from build123d import *

# Parameters (mm, degrees)
BOSS_EXTRUDE2_DEPTH                           = 9
CUT_EXTRUDE3_DEPTH                            = 37.794697197
CUT_EXTRUDE3_DEPTH_BACK                       = 29.526
SKETCH3_W                                     = 7.1119396
SKETCH3_H                                     = 8
SKETCH3_W_2                                   = 47.10835744
BOSS_EXTRUDE3_DEPTH                           = 14.032
BOSS_EXTRUDE3_DEPTH_BACK                      = 1
BOSS_EXTRUDE4_START                           = 2.072367721
BOSS_EXTRUDE4_DEPTH                           = 6.927632279
CSK_FOR_3_FLAT_HEAD_SOCKET_CAP_SCREW1_A_COUNT = 2
CSK_FOR_3_FLAT_HEAD_SOCKET_CAP_SCREW1_A_PITCH = 19.290792


# Read off the part's stored shape, not the designer's step: Boss-Extrude4
with BuildPart() as part:
    # Sketch2 → Boss-Extrude2 (new body)
    with BuildSketch(Plane.XY):
        Polygon((-9.096510891, -26.330282843), (-9.701316376, -34.435752293), (-2.609093023, -34.964952435), (-3.061940834, -41.033918716), (-2.048641284, -41.109525962), (-1.973042695, -40.096342438), (0.937582862, -1.088781958), (1.013181451, -0.075598434), (0, 0), (-0.567761002, -7.60900747), (-7.660098307, -7.079798826), (-8.264903605, -15.18526578), (-1.1725663, -15.714474425), (-2.004173586, -26.859491487), align=None)
    extrude(amount=BOSS_EXTRUDE2_DEPTH)

    # Sketch3 → Cut-Extrude3 (cut, two sides: drawn at the far end of the back side and taken through both)
    with BuildSketch(Plane(origin=(-2.608979071, -34.964960937, 0), x_dir=(0.9972277257028987, -0.07441010072177218, 0), z_dir=(-0.07441010072177218, -0.9972277257028987, 0)).offset(-CUT_EXTRUDE3_DEPTH_BACK)):
        with Locations((-3.556084069, 5)):
            Rectangle(SKETCH3_W, SKETCH3_H)
        with Locations((-30.666232589, 5)):
            Rectangle(SKETCH3_W_2, SKETCH3_H)
    extrude(amount=CUT_EXTRUDE3_DEPTH + CUT_EXTRUDE3_DEPTH_BACK, mode=Mode.SUBTRACT)

    # Sketch4 → Boss-Extrude3 (add, two sides: drawn at the far end of the back side and taken through both)
    with BuildSketch(Plane(origin=(1.013183369, -0.075600662, 0), x_dir=(0, 0, -1), z_dir=(0.9972277257028997, -0.07441010072175744, 0)).offset(-BOSS_EXTRUDE3_DEPTH_BACK)):
        Polygon((-9, -41.147998684), (-9, 2.079e-06), (-10, 0), (-10, -41.147998684), align=None)
    extrude(amount=BOSS_EXTRUDE3_DEPTH + BOSS_EXTRUDE3_DEPTH_BACK)

    # Boss-Extrude4 outline → Boss-Extrude4 (add)
    with BuildSketch(Plane.XY.offset(BOSS_EXTRUDE4_START)):
        Polygon((-0.054187906, -41.258346009), (3.007638975, -0.22441879), (1.013181451, -0.075598434), (0.937582862, -1.088781958), (-1.973042695, -40.096342438), (-2.048641284, -41.109525962), align=None)
    extrude(amount=BOSS_EXTRUDE4_DEPTH)

    # Sketch6 → CSK for _3 Flat Head Socket Cap Screw1 (revolve, cut)
    with BuildSketch(Plane(origin=(-4.41257913, -11.346475453, 1), x_dir=(0, -1, 0), z_dir=(1, 0, 0))):
        Polygon((0, 0), (0, 1), (1.397, 1), (1.397, 1.694722738), (2.8702, 0), align=None)
    csk_for_3_flat_head_socket_cap_screw1 = revolve(axis=Axis((-4.41257913, -11.346475453, 7.35), (0, 0, -1)), mode=Mode.SUBTRACT)

    # CSK for _3 Flat Head Socket Cap Screw1 a: CSK for _3 Flat Head Socket Cap Screw1 ×2
    with Locations(*[Vector(-0.07441010072177331, -0.9972277257028986, 0) * (i * CSK_FOR_3_FLAT_HEAD_SOCKET_CAP_SCREW1_A_PITCH) for i in range(1, CSK_FOR_3_FLAT_HEAD_SOCKET_CAP_SCREW1_A_COUNT)]):
        add(csk_for_3_flat_head_socket_cap_screw1, mode=Mode.SUBTRACT)


solid = part.part
Build history of the part. All positions in model axes, mm. A direction names the side the tool comes from. Coordinates: 2 decimals unless noted, no trailing zeros. Order: outer loops, then holes, each group sorted by start corner. A loop starts at its lowest first (then second) coordinate and runs counter-clockwise, first axis right, second up. Notation, with made-up numbers: (71, 4.5) - (96, 4.5) arc R15 cw to (96, 33.5) - close; hole circle Ø7 at (27.25, 36.5). An arc over 180 degrees is marked (long way). Put each result on its own line as item: value.
1. Probe line 1 along Z through (x, y) = (8.5, -9); line 2 along Y through (x, z) = (-6.5, 0.5); line 3 along X through (y, z) = (-8, 4.25). List the from-to ranges inside material, lowest first. Write a range as [from, to].
Answer sheet:
line 1: z = [9, 10]
line 2: y = [-34.67, -32.93], [-28.24, -26.52], [-15.32, -12.6], [-10.09, -7.17]
line 3: x = [-0.6, 2.43]
2. Saw through at D-D (x = 13). Write the cut outline in (y, z).
Answer sheet:
outline: (-28.01, 9) - (-0.97, 9) - (-0.97, 10) - (-28.01, 10) - close
3. Drop flat-ended pins along their axis: P1, Ø4, axis at x = -0.5, y = -11, coming from the -Z side; P2, Ø3, axis at y = -10, z = 9, coming from the -X side; P3, Ø1.5, axis at y = -37.5, z = 2.5, coming from the -X side; P4, Ø4, axis at x = -7, y = -33, coming from the +Z side. Give the stop position or say it passes through.
Answer sheet:
P1: stops at z = 0
P2: stops at x = -0.86
P3: stops at x = -2.85
P4: stops at z = 1
4. Tool access for faces 1 (the face through (-4.097, -7.346, 0.479)), 2 (the face through (-4.74, -15.45, 0.48)), 3 (the face through (-4, -33, 1)): list every direction of +Z, -Z, +X, -X, +Y, -Y with a clear straight run to the whole face (end or side of a thin tool).
Answer sheet:
face 1: +Z, -Z, +Y
face 2: +Z, -Z, -X
face 3: +Z, -X, +Y
5. Pull direction Y, two halves, no side cores. Call faces 4 (the face through (-5.5, -26.6, 0.5)), 5 (the face through (1.455, -21.029, 5.488)), 6 (the face through (7, -21, 9)): pulls with the +Y half, pulls with the -Y half, needs draft (parallel to the pull), parting line crosses it, or undercut.
Answer sheet:
face 4: undercut
face 5: pulls with the -Y half
face 6: needs draft
